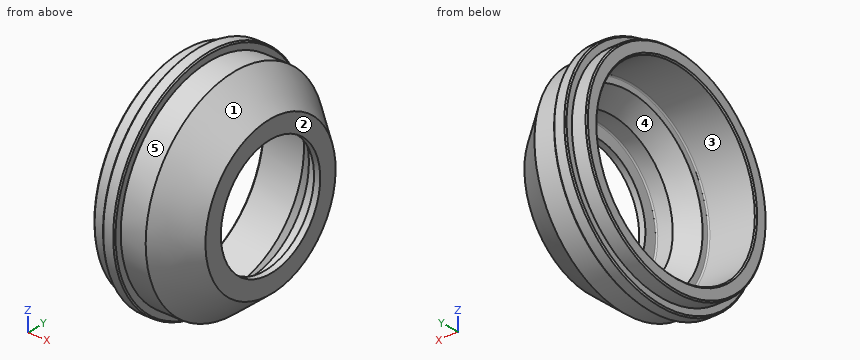
from build123d import *

# Parameters (mm, degrees)
ZAOKR_GLENIE1_R  = 1
ZAOKR_GLENIE2_R  = 1
SFAZOWANIE1_SIZE = 1


with BuildPart() as part:
    # Szkic1 → Obrót1 (revolve)
    with BuildSketch(Plane.XY, mode=Mode.PRIVATE) as obr_t1_sk:
        Polygon((70, 47), (65, 47), (65, 57.5), (52, 57.5), (38, 69.247394836), (38, 75), (0, 75), (0, 85), (12, 85), (12, 91), (22, 91), (22, 85), (42, 85), (70, 61.505210327), align=None)
    revolve(obr_t1_sk.sketch.rotate(Axis((0, 0, 0), (1, 0, 0)), 90), axis=Axis((0, 0, 0), (1, 0, 0)))  # turned: the seam where the file's is

    # Zaokrąglenie1
    zaokr_glenie1_edges = [part.edges().sort_by_distance(p)[0] for p in [
        (65, 0, -57.5),
    ]]
    fillet(zaokr_glenie1_edges, radius=ZAOKR_GLENIE1_R)

    # Zaokrąglenie2
    zaokr_glenie2_edges = [part.edges().sort_by_distance(p)[0] for p in [
        (38, 0, -75),
    ]]
    fillet(zaokr_glenie2_edges, radius=ZAOKR_GLENIE2_R)

    # Sfazowanie1
    sfazowanie1_edges = [part.edges().sort_by_distance(p)[0] for p in [
        (22, 0, -91),
        (12, 0, -91),
        (0, 0, -85),
        (0, 0, -75),
    ]]
    chamfer(sfazowanie1_edges, length=SFAZOWANIE1_SIZE)


solid = part.part
For this review, take the finished solid that the model builds, in its own axes (mm). Face numbers are marked on the shaded views. A direction names the side the tool comes from. Round coordinates to 2 decimals unless told otherwise and drop trailing zeros. Write each loop counter-clockwise with the first axis right and the second up, starting at its lowest first coordinate (ties: lowest second). Pieces come first, ordered by that corner, then holes. Notation, with made-up numbers: (47.5, 40.5) -> (101.5, 40.5) arc R16 cw to (101.5, 67.5) -> close; hole circle Ø4 at (5, 5.25). An arc over 180 degrees is marked (long way). Put each result on its own line as item: value.
Q1. The part is to be moulded in two halves that separate along Y. For the marked faces 1, 2 and 3, say which applies: released by +Y, released by -Y, zero draft, split by the parting line, or undercut.
Determined:
face 1: split by the parting line
face 2: zero draft
face 3: undercut
Q2. Consider section B-B on x = 57. State the section outline as (y, z) points, and give its area (3 significant figures).
Determined:
outline: circle Ø144.83 at (0, 0); hole circle Ø115 at (0, 0)
area: 6,090 mm^2
Q3. To check wall thickness, follow L1, parallel to Y at x = 18, z = 0; L2, parallel to Z at x = 36.5, y = 0.5; L3, parallel to X at y = 68, z = 57. State the ranges of each line that lie inside material, in increasing order. Write a range as [from, to].
Determined:
L1: y = [-91, -75], [75, 91]
L2: z = [-85, -75], [75, 85]
L3: x = [12, 22]
Q4. Consider section A-A on x = 17. State the section outline as (y, z) points, and give its area (3 significant figures).
Determined:
outline: circle Ø182 at (0, 0); hole circle Ø150 at (0, 0)
area: 8,340 mm^2
Q5. Clearance check with flat-ended pins moving along their axes: pin 1 Ø6 at (x, y) = (40, 69.5) entering from -Z; pin 2 Ø10 at (x, z) = (28.5, 18) entering from +Y; pin 3 Ø4 at (x, z) = (21, 47.5) entering from -Y. State where each tip first meets the part, or that it passes through.
Determined:
pin 1: stops at z = -52.94
pin 2: stops at y = 84
pin 3: stops at y = -78.81
Q6. Machinability: for the marked faces 4 and 5, which of the approach directions +Z, -Z, +X, -X, +Y, -Y give a long, thin tool a straight path to every point of the face, cutting with its end or side? Answer none if there is none.
Determined:
face 4: -X
face 5: +X
